The listing builds one solid part. Answer for the finished solid, in the listing's coordinates (mm). Face numbers are marked on the shaded views. Give positions to 0.01 mm unless a question says otherwise; leave off trailing zeros. Write each loop counter-clockwise with the first axis right and the second up, starting at its lowest first coordinate (ties: lowest second). Pieces come first, ordered by that corner, then holes. Notation, with made-up numbers: (23, -8.75) - (71, -8.75) arc R12 cw to (71, -1.75) - close; hole circle Ø1 at (14, 37). An arc over 180 degrees is marked (long way). Write each question's results on one line, items separated by ' | '. Start each with the question number.
Q1. Section C-C (y = 4) is taken. Determine the outline of the cut face in (x, z).
Q2. For a pull along Z with two mould halves and no side action, classify the marked faces 1, 2, 3 and 4 as pulls with the +Z half, pulls with the -Z half, needs draft (parallel to the pull), parting line crosses it, or undercut.
Q3. Section D-D (y = 1.5) is taken. Determine the outline of the cut face in (x, z), plus the area to 3 significant figures.
Q4. A flat-ended cylindrical pin translates along its axis: pin 1 Ø2.5 at (x, y) = (4, 4) entering from -Z. Find the tip coordinate at first contact, or state that the pin passes through.
Q5. Find the intervals of material crossed by probe 1 along Y at (x, z) = (4, 1); probe 2 along X at (y, z) = (4.25, 0); probe 3 along Z at (x, y) = (-5.75, 6), in increasing order.
Q6. Section A-A (z = 0) is taken. Determine the outline of the cut face in (x, y), plus the area to 3 significant figures.
Q7. Section B-B (x = -4) is taken. Determine the outline of the cut face in (y, z), plus the area to 3 significant figures.
```python
from build123d import *

# Parameters (mm, degrees)
SKETCH_1_W             = 16
SKETCH_1_H             = 8
EXTRUDE_1_DEPTH        = 8
HOLE_WIZARD_M4_2_D     = 3.3
HOLE_WIZARD_M4_2_DEPTH = 11.6
HOLE_WIZARD_M4_2_TIP   = 0.991420021
FILLET_1_R             = 1
SKETCH_7_R             = 2
CUT_EXTRUDE_1_DEPTH    = 10


with BuildPart() as part:
    # 草图1 → 凸台-拉伸1 (new body)
    with BuildSketch(Plane(origin=(0, 0, 0), x_dir=(1, 0, 0), z_dir=(0, 1, 0))):
        Rectangle(SKETCH_1_W, SKETCH_1_H)
    extrude(amount=EXTRUDE_1_DEPTH)

    # M4 螺纹孔2
    with Locations(Plane.XY.offset(4)):
        with Locations((4, 4)):
            Hole(HOLE_WIZARD_M4_2_D / 2, depth=HOLE_WIZARD_M4_2_DEPTH)
            with Locations((0, 0, -(HOLE_WIZARD_M4_2_DEPTH + HOLE_WIZARD_M4_2_TIP / 2))):  # 118° drill point
                Cone(0, HOLE_WIZARD_M4_2_D / 2, HOLE_WIZARD_M4_2_TIP, mode=Mode.SUBTRACT)

    # 圆角1
    fillet_1_edges = [part.edges().sort_by_distance(p)[0] for p in [
        (8, 4, 4),
        (-8, 4, 4),
        (-8, 4, -4),
        (8, 4, -4),
    ]]
    fillet(fillet_1_edges, radius=FILLET_1_R)

    # 草图7 → 切除-拉伸1 (cut)
    with BuildSketch(Plane(origin=(0, 8, 0), x_dir=(1, 0, 0), z_dir=(0, 1, 0))):
        with Locations(Location((-4, 0, 0), (0, 0, 270))):
            Circle(SKETCH_7_R)
    extrude(amount=-CUT_EXTRUDE_1_DEPTH, mode=Mode.SUBTRACT)


solid = part.part
```
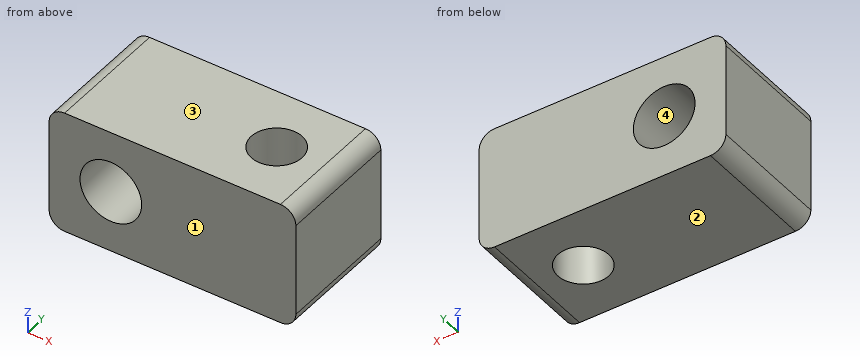
Answers below:
1) outline: (-8, -3) arc R1 ccw to (-7, -4) - (2.35, -4) - (2.35, 4) - (-7, 4) arc R1 ccw to (-8, 3) - close; (5.65, -4) - (7, -4) arc R1 ccw to (8, -3) - (8, 3) arc R1 ccw to (7, 4) - (5.65, 4) - close; hole circle Ø4 at (-4, 0)
2) face 1: needs draft | face 2: pulls with the -Z half | face 3: pulls with the +Z half | face 4: undercut
3) outline: (-8, -3) arc R1 ccw to (-7, -4) - (7, -4) arc R1 ccw to (8, -3) - (8, 3) arc R1 ccw to (7, 4) - (-7, 4) arc R1 ccw to (-8, 3) - close; hole circle Ø4 at (-4, 0) | area: 115 mm2
4) pin 1: passes through
5) probe 1: y = 0 to 2.35, 5.65 to 8 | probe 2: x = -8 to -6, -2 to 2.37, 5.63 to 8 | probe 3: z = -4 to -0.97, 0.97 to 4
6) outline: (-8, 0) - (-6, 0) - (-6, 8) - (-8, 8) - close; (-2, 0) - (8, 0) - (8, 8) - (-2, 8) - close; hole circle Ø3.3 at (4, 4) | area: 87.4 mm2
7) outline: (0, -4) - (8, -4) - (8, -2) - (0, -2) - close; (0, 2) - (8, 2) - (8, 4) - (0, 4) - close | area: 32.0 mm2
